Check sheet for the modelled part. Datum: model origin and axes. Units: mm. Round coordinates to 2 decimals unless told otherwise and drop trailing zeros. Write each loop counter-clockwise with the first axis right and the second up, starting at its lowest first coordinate (ties: lowest second). Pieces come first, ordered by that corner, then holes.
Item 1: Go/stop test with flat-tipped pins: pin 1 Ø10 at (x, z) = (21.5, 13) entering from +Y; pin 2 Ø3 at (x, y) = (5.5, -11) entering from +Z; pin 3 Ø10 at (x, y) = (19.5, -20.5) entering from +Z. Record where each tip stops, or that it passes through.
Item 2: Material ranges on line 1 (Z direction, x = 24, y = 19); line 2 (Z direction, x = 16, y = 21); line 3 (Y direction, x = 8.5, z = 19), recorded low to high.
Item 3: Cross-section at A-A on z = 38. Enter the section's corners in (x, y), plus the area to 3 significant figures.
Item 4: Cross-section at B-B on y = 46. Enter the section's corners in (x, z) (3 decimals), plus the area to 3 significant figures.
from build123d import *

# Parameters (mm, degrees)
F1_DEPTH    = 25.4
F2_T1_DEPTH = 238.6235911332
F3_SIZE2    = 7.62
F3_SIZE     = 12.7


# Not quite as in the source:
# - a fillet or chamfer that OpenCascade refuses, or shapes differently, is made with other operations: its cross-section is extruded or revolved along the edge and cut away or added


with BuildPart() as f1:
    # F0 (on Right) → F1 (new body)
    with BuildSketch(Plane.YZ):
        Polygon((-44.9345260859, 0), (0, 0), (60.6710910797, 17.4429379404), (10.2382460609, 44.3657338619), (-54.0351904929, 21.4244797826), align=None)
    extrude(amount=F1_DEPTH)

    # F2: fillet of radius 48.2774474346 on 1 edges, made by hand

    # F2_s2 → F2_t1 (cut)
    with BuildSketch(Plane.YZ.offset(-106.6117955666)):
        with BuildLine():
            add(Edge.make_bspline(
                [(-44.9345260859, 0), (-39.4692303476, 26.6235388421), (-13.8721919012, 35.7599440845)],
                knots=[0, 0, 0, 1, 1, 1], degree=2, weights=[1, 1, 1]))
            Line((-13.8721919012, 35.7599440845), (-54.0351904929, 21.4244797826))
            Line((-54.0351904929, 21.4244797826), (-44.9345260859, 0))
        make_face()
    extrude(amount=F2_T1_DEPTH, mode=Mode.SUBTRACT)

    # F3
    f3_edges = [f1.edges().sort_by_distance(p)[0] for p in [
        (12.7, 10.238246, 44.365734),
    ]]
    f3_side = f1.faces().sort_by_distance((12.7, -1.816973, 40.062839))[0]
    chamfer(f3_edges, length=F3_SIZE, length2=F3_SIZE2, reference=f3_side)


solid = f1.part
Response values:
1. pin 1: stops at y = 60.67
1. pin 2: stops at z = 37.32
1. pin 3: stops at z = 35.15
2. line 1: z = 5.46 to 39.69
2. line 2: z = 6.04 to 38.62
2. line 3: y = -36.99 to 57.75
3. outline: (0, -7.6) - (25.4, -7.6) - (25.4, 22.16) - (0, 22.16) - close
3. area: 756 mm2
4. outline: (0, 13.225) - (25.4, 13.225) - (25.4, 25.275) - (0, 25.275) - close
4. area: 306 mm2
